from build123d import *

# Parameters (mm, degrees)
SKETCH1_R           = 87.5
BOSS_EXTRUDE1_DEPTH = 9.5
SKETCH2_R           = 87.5
SKETCH2_R_2         = 71.9
CUT_EXTRUDE1_DEPTH  = 16.5
SKETCH3_R           = 45.4
CUT_EXTRUDE2_DEPTH  = 16.5
CHAMFER1_SIZE       = 15
CHAMFER1_SIZE2      = 8.660254038
FILLET1_R           = 4
CUT_EXTRUDE3_DEPTH  = 126.193849689
SKETCH6_R           = 1.75
CUT_EXTRUDE4_DEPTH  = 126.193849689


# Read off the part's stored shape, not the designer's step: Shell1
with BuildPart() as part:
    # Sketch1 → Boss-Extrude1 (new, symmetric)
    with BuildSketch(Plane.XY):
        Circle(SKETCH1_R)
    extrude(amount=BOSS_EXTRUDE1_DEPTH, both=True)

    # Sketch2 → Cut-Extrude1 (cut)
    with BuildSketch(Plane.XY.offset(9.5)):
        Circle(SKETCH2_R)
        Circle(SKETCH2_R_2, mode=Mode.SUBTRACT)
    extrude(amount=-CUT_EXTRUDE1_DEPTH, mode=Mode.SUBTRACT)

    # Sketch3 → Cut-Extrude2 (cut)
    with BuildSketch(Plane.XY.offset(9.5)):
        Circle(SKETCH3_R)
    extrude(amount=-CUT_EXTRUDE2_DEPTH, mode=Mode.SUBTRACT)

    # Chamfer1
    chamfer1_edges = [part.edges().sort_by_distance(p)[0] for p in [
        (-71.9, 0, 9.5),
    ]]
    chamfer1_side = [part.faces().sort_by_distance(p)[0] for p in [
        (-71.9, 0, 1.25),
    ]]
    chamfer(chamfer1_edges, length=CHAMFER1_SIZE, length2=CHAMFER1_SIZE2, reference=chamfer1_side[0])

    # Fillet1
    fillet1_edges = [part.edges().sort_by_distance(p)[0] for p in [
        (-45.4, 0, 9.5),
        (-63.239745962, 0, 9.5),
    ]]
    fillet(fillet1_edges, radius=FILLET1_R)

    # Shell1 outline → Shell1 (revolve, cut)
    with BuildSketch(Plane.XZ):
        with BuildLine():
            Line((47.9, -9.5), (69.4, -9.5))
            Line((69.4, -9.5), (69.4, -6.169872981))
            Line((69.4, -6.169872981), (62.229382991, 6.25))
            ThreePointArc((62.229382991, 6.25), (61.680344885, 6.799038106), (60.930344885, 7))
            Line((60.930344885, 7), (49.4, 7))
            ThreePointArc((49.4, 7), (48.339339828, 6.560660172), (47.9, 5.5))
            Line((47.9, 5.5), (47.9, -9.5))
        make_face()
    revolve(axis=Axis((0, 0, 0), (0, 0, 1)), mode=Mode.SUBTRACT)

    # Sketch5 → Cut-Extrude3 (cut, through all)
    with BuildSketch(Plane(origin=(0, 0, -9.5), x_dir=(-1, 0, 0), z_dir=(0, 0, -1))):
        with BuildLine():
            ThreePointArc((-13.8, 18.4), (-23, 0), (-13.8, -18.4))
            ThreePointArc((-13.8, -18.4), (-9.6, -17.8), (-10.2, -13.6))
            ThreePointArc((-10.2, -13.6), (-17, 0), (-10.2, 13.6))
            ThreePointArc((-10.2, 13.6), (-9.6, 17.8), (-13.8, 18.4))
        make_face()
    cut_extrude3 = extrude(amount=-CUT_EXTRUDE3_DEPTH, mode=Mode.SUBTRACT)

    # Mirror1: Cut-Extrude3 across plane
    add(cut_extrude3.mirror(Plane(origin=(0, 0, 0), x_dir=(0, 0, 1), z_dir=(1, 0, 0))), mode=Mode.SUBTRACT)

    # Sketch6 → Cut-Extrude4 (cut, through all)
    with BuildSketch(Plane.XY.offset(9.5)):
        with Locations((-55.1, 0)):
            Circle(SKETCH6_R)
    cut_extrude4 = extrude(amount=-CUT_EXTRUDE4_DEPTH, mode=Mode.SUBTRACT)

    # Mirror2: Cut-Extrude4 across plane
    add(cut_extrude4.mirror(Plane(origin=(0, 0, 0), x_dir=(0, 0, 1), z_dir=(1, 0, 0))), mode=Mode.SUBTRACT)


solid = part.part
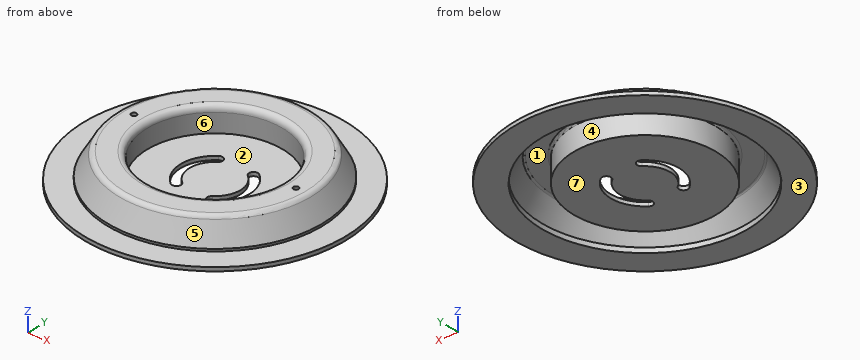
The model under review builds one solid part; all positions refer to its coordinate system, in mm. Face numbers are marked on the shaded views. A direction names the side the tool comes from. Round coordinates to 2 decimals unless told otherwise and drop trailing zeros. Order: outer loops, then holes, each group sorted by start corner. A loop starts at its lowest first (then second) coordinate and runs counter-clockwise, first axis right, second up. Notation, with made-up numbers: (39.5, 43) -> (74.5, 43) arc R10 ccw to (74.5, 59) -> close; hole circle Ø6 at (24, 75.5). An arc over 180 degrees is marked (long way). Use CSV: the item, a comma, the result in double quotes. Start each with the question number.
(1) Wall thickness on probe 1 along X at (y, z) = (-3.5, -7.75); probe 2 along Y at (x, z) = (0, 3.25); probe 3 along X at (y, z) = (1.5, -1.75): over which ranges is each line inside the solid? List them lowest first. Write a range as from..to.
(2) Consider section B-B on y = -11. State how many separate pieces and enclosed holes the cut face has, and give its area (3 significant figures).
(3) Insertion check: pin 1 (10 mm diameter, centred on x = -10, y = -45.5, fed in from +Z); pin 2 (1.5 mm diameter, centred on y = 53, z = -0.5, fed in from -X); pin 3 (5 mm diameter, centred on x = -33.5, z = -7.5, fed in from +Y); pin 4 (1.5 mm diameter, centred on x = -12, z = -1.5, fed in from -Y). Each pin has a flat end and moves straight along its axis. Give the tip position at first contact, or say it passes through.
(4) Mouldability with a two-part tool opening along X and no side actions: class the marked faces 4, 5, 6 and 7 as pulls with the +X half, pulls with the -X half, needs draft (parallel to the pull), parting line crosses it, or undercut.
(5) Consider section C-C on x = -74. Write out the cut boundary in (y, z), and give its area (3 significant figures).
(6) Consider section A-A on z = -1.25. Write out the cut boundary in (x, y).
(7) Tool access review of the marked faces 1, 2 and 3: name each direction out of +Z, -Z, +X, -X, +Y, -Y from which nothing blocks a thin tool from reaching the whole face with its end or side.
Responses:
1,probe 1,"-87.43..-69.31, -47.77..-22.73, -16.64..16.64, 22.73..47.77, 69.31..87.43"
1,probe 2,"-66.85..-63.96, -47.9..-45.4, 45.4..47.9, 63.96..66.85"
1,probe 3,"-69.72..-66.83, -47.88..-45.38, 45.38..47.88, 66.83..69.72"
2,separate pieces,"3"
2,enclosed holes,"0"
2,area,"529 mm²"
3,pin 1,"z = 9.5"
3,pin 2,"x = -45.31"
3,pin 3,"y = 81.82"
3,pin 4,"y = -69.01"
4,face 4,"undercut"
4,face 5,"parting line crosses it"
4,face 6,"undercut"
4,face 7,"needs draft"
5,outline,"(-46.69, -9.5) -> (46.69, -9.5) -> (46.69, -7) -> (-46.69, -7) -> close"
5,area,"233 mm²"
6,outline,"circle Ø138.89 at (0, 0); circle Ø95.8 at (0, 0); hole circle Ø133.12 at (0, 0); hole circle Ø90.8 at (0, 0)"
7,face 1,"-Z"
7,face 2,"+Z"
7,face 3,"-Z, +X, -X, +Y, -Y"
